Part model, mm, in its own coordinate system. A direction names the side the tool comes from. Round coordinates to 2 decimals unless told otherwise and drop trailing zeros. Write each loop counter-clockwise with the first axis right and the second up, starting at its lowest first coordinate (ties: lowest second). Pieces come first, ordered by that corner, then holes. Notation, with made-up numbers: (26.5, 26.25) -> (84.5, 26.25) arc R9 ccw to (84.5, 34.25) -> close; hole circle Ø11 at (-16, 20). An arc over 180 degrees is marked (long way). Return JSON: item names as keys, results as strings. Group by question number.
(1) Drill centre lines: L1, parallel to Y at x = -0.5, z = 1.25; L2, parallel to X at y = -5, z = 3.25; L3, parallel to Z at x = 0.25, y = -2.25. Where is each one in solid material? Low to high. Write a range as from..to.
(2) Tool access for faces 4 (the flat face through (0, 0, 25)), 5 (the flat face through (0, 0, 23.5)): list every direction of +Z, -Z, +X, -X, +Y, -Y with a clear straight run to the whole face (end or side of a thin tool).
(3) Saw through at A-A (z = 13.5). List the corners of the cut face in (x, y).
(4) Mould opens along Y. For faces 1 (the conical face through (9.925, 3.126, 11.877)), 2 (the conical face through (-1.93, -8.7, 11.72)), 3 (the flat face through (0.9, -11.1, 0)) say: +Y half, -Y half, draft (parallel to the pull), parting line (faces both ways), or undercut.
(5) Drop flat-ended pins along their axis: pin 1 Ø5 at (y, z) = (-7, 21) entering from +X; pin 2 Ø8 at (x, y) = (-6, -2.5) entering from +Z; pin 3 Ø3 at (x, z) = (0, 22) entering from +Y. Give the stop position or say it passes through.
from build123d import *

# Parameters (mm, degrees)
F0_R     = 12.5
F1_DEPTH = 25
F1_TAPER = 10
F2_R     = 7
F3_T     = -1.5


with BuildPart() as f1:
    # F0 (on Top) → F1 (new body)
    with BuildSketch(Plane.XY):
        Circle(F0_R)
    extrude(amount=F1_DEPTH, taper=F1_TAPER)

    # F2
    f2_edges = [f1.edges().sort_by_distance(p)[0] for p in [
        (-8.091825, 0, 25),
    ]]
    fillet(f2_edges, radius=F2_R)

    # F3
    f3_openings = [f1.faces().sort_by_distance(p)[0] for p in [
        (0, 0, 0),
    ]]
    offset(amount=F3_T, openings=f3_openings)


solid = f1.part
Computed values:
{
 "1": {"L1": "-12.27..-10.74, 10.74..12.27", "L2": "-10.83..-9.12, 9.12..10.83", "L3": "23.5..25"},
 "2": {"face 4": "+Z, +X, -X, +Y, -Y", "face 5": "-Z"},
 "3": {"outline": "circle Ø20.24 at (0, 0); hole circle Ø17.19 at (0, 0)"},
 "4": {"face 1": "parting line", "face 2": "undercut", "face 3": "draft"},
 "5": {"pin 1": "x = 7.59", "pin 2": "z = 24.99", "pin 3": "y = 8.76"}
}
